Check sheet for the modelled part. Datum: model origin and axes. Units: mm. Face numbers are marked on the shaded views. A direction names the side the tool comes from. Give positions to 0.01 mm unless a question says otherwise; leave off trailing zeros. Loops run counter-clockwise (first coordinate to the right, second up) from the corner with the lowest first, then second, coordinate; pieces in that order, holes last. Notation, with made-up numbers: (39.5, 35.25) - (51.5, 35.25) arc R12 ccw to (51.5, 57.25) - close; hole circle Ø8 at (-23, -3.5). An arc over 180 degrees is marked (long way). Use one line per item in the form item = value.
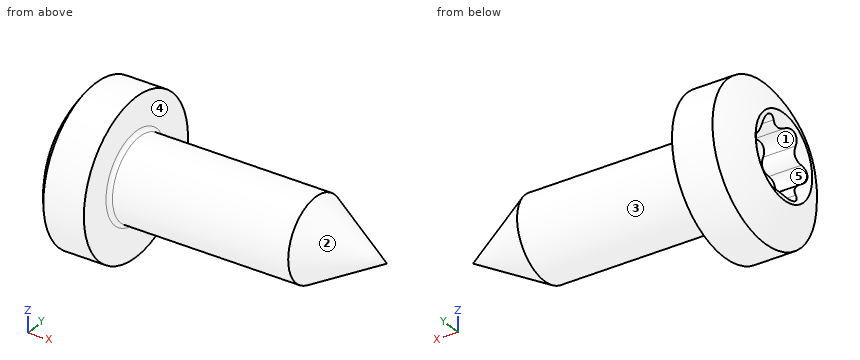
from build123d import *

# Parameters (mm, degrees)
CUT_EXTRUDE_1_REACH = 8.451
FILLET_1_R          = 0.2


with BuildPart() as part:
    # 草图2 → 旋转1 (revolve)
    with BuildSketch(Plane.XY):
        with BuildLine():
            Line((0, 0), (0, 4))
            Line((0, 4), (-2.097282132, 4))
            ThreePointArc((-2.097282132, 4), (-2.672376759, 3.126707508), (-3.1, 2.1725))
            Line((-3.1, 2.1725), (-3.1, 0))
            Line((-3.1, 0), (0, 0))
        make_face()
    revolve(axis=Axis((0, 0, 0), (-1, 0, 0)))

    # 草图3 → 切除-拉伸1 (cut, up to next)
    with BuildSketch(Plane(origin=(0, 0, 0), x_dir=(0, 0, -1), z_dir=(1, 0, 0)), mode=Mode.PRIVATE) as cut_extrude_1_sk1:
        with BuildLine():
            ThreePointArc((-0.476528859, 1.6908006), (0, 1.975), (0.476528859, 1.6908006))
            ThreePointArc((0.476528859, 1.6908006), (0.79, 1.368320138), (1.226011842, 1.258086397))
            ThreePointArc((1.226011842, 1.258086397), (1.710400172, 0.9875), (1.702540702, 0.432714202))
            ThreePointArc((1.702540702, 0.432714202), (1.58, 0), (1.702540702, -0.432714202))
            ThreePointArc((1.702540702, -0.432714202), (1.710400172, -0.9875), (1.226011842, -1.258086397))
            ThreePointArc((1.226011842, -1.258086397), (0.79, -1.368320138), (0.476528859, -1.6908006))
            ThreePointArc((0.476528859, -1.6908006), (0, -1.975), (-0.476528859, -1.6908006))
            ThreePointArc((-0.476528859, -1.6908006), (-0.79, -1.368320138), (-1.226011842, -1.258086397))
            ThreePointArc((-1.226011842, -1.258086397), (-1.710400172, -0.9875), (-1.702540702, -0.432714202))
            ThreePointArc((-1.702540702, -0.432714202), (-1.58, 0), (-1.702540702, 0.432714202))
            ThreePointArc((-1.702540702, 0.432714202), (-1.710400172, 0.9875), (-1.226011842, 1.258086397))
            ThreePointArc((-1.226011842, 1.258086397), (-0.79, 1.368320138), (-0.476528859, 1.6908006))
        make_face()
    cut_extrude_1_tool1 = extrude(cut_extrude_1_sk1.sketch, amount=-CUT_EXTRUDE_1_REACH, mode=Mode.PRIVATE) & part.part
    add(cut_extrude_1_tool1.solids().sort_by_distance((0, 0, 0))[0], mode=Mode.SUBTRACT)

    # 草图4 → 旋转2 (revolve)
    with BuildSketch(Plane.XY, mode=Mode.PRIVATE) as revolve_2_sk:
        Polygon((0, 1.975), (-1.3, 1.975), (-0.159733218, 0), (0, 0), align=None)
    revolve(revolve_2_sk.sketch.rotate(Axis((0, 0, 0), (-1, 0, 0)), 270), axis=Axis((0, 0, 0), (-1, 0, 0)))

    # 切除-拉伸2 cone 1 section (through the dimple's axis) → 切除-拉伸2 (revolve, cut)
    with BuildSketch(Plane(origin=(-3.1, 0, 0), x_dir=(0, 0, 1), z_dir=(0, 1, 0))):
        Polygon((0, 0), (2.1725, 0), (0, 1.25429346), align=None)
    revolve(axis=Axis((-3.1, 0, 0), (1, 0, 0)), mode=Mode.SUBTRACT)

    # 草图6 → 旋转3 (revolve)
    with BuildSketch(Plane.XY, mode=Mode.PRIVATE) as revolve_3_sk:
        Polygon((0, 2.1), (9.3, 2.1), (13, 0), (0, 0), align=None)
    revolve(revolve_3_sk.sketch.rotate(Axis((0, 0, 0), (-1, 0, 0)), 164.260244237), axis=Axis((0, 0, 0), (-1, 0, 0)))

    # 圆角1
    fillet_1_edges = [part.edges().sort_by_distance(p)[0] for p in [
        (0, 2.021257882, 0.569663562),
    ]]
    fillet(fillet_1_edges, radius=FILLET_1_R)


solid = part.part
Item 1: Section check C-C on y = 2.5. Record the boundary of the cut face in (x, z), then the cut area to 3 significant figures.
Answer block:
outline = (-2.1, -3.12) - (0, -3.12) - (0, 3.12) - (-2.1, 3.12) arc R6 ccw to start
area = 16.8 mm2
Item 2: Section check B-B on x = 1.5. Record the boundary of the cut face in (y, z).
Answer block:
outline = circle Ø4.2 at (0, 0)
Item 3: Mould release check, pull along Z, two halves, no side actions. Record for the marked faces 3, 4 and 5: released by +Z, released by -Z, zero draft, split by the parting line, or undercut.
Answer block:
face_3 = split by the parting line
face_4 = zero draft
face_5 = undercut
Item 4: Section check D-D on x = 10.5. Record the boundary of the cut face in (y, z), then the cut area to 3 significant figures.
Answer block:
outline = circle Ø2.84 at (0, 0)
area = 6.33 mm2
Item 5: Gauge pin test, flat ends, axial feed: P1, Ø4, axis at x = 4, y = 2.5, coming from the +Z side; P2, Ø1, axis at x = 0, z = -1, coming from the +Y side. Record the tip position at first contact, or that the pin passes through.
Answer block:
P1 = 2.04
P2 = 3.97
Item 6: Section check A-A on z = -2.75. Record the boundary of the cut face in (x, y).
Answer block:
outline = (-2.1, -2.9) - (0, -2.9) - (0, 2.9) - (-2.1, 2.9) arc R5.89 ccw to start
Item 7: Thickness scan on L1, parallel to Z at x = 2.75, y = 0; L2, parallel to Z at x = -1.75, y = 0.5; L3, parallel to Z at x = 7.25, y = 1. Record the ranges inside material, lowest first.
Answer block:
L1 = -2.1 to 2.1
L2 = -3.97 to -1.74, 1.74 to 3.97
L3 = -1.85 to 1.85
Item 8: Access from +Z, -Z, +X, -X, +Y, -Y to the whole of each face (thin tool, end or side, straight path). Record for the marked faces 1 and 2.
Answer block:
face_1 = -X
face_2 = +X
